Source: CAD feature listing. Evaluate the final solid. Frame: model axes, mm. A direction names the side the tool comes from. Give positions to 0.01 mm unless a question says otherwise; leave off trailing zeros. Order: outer loops, then holes, each group sorted by start corner. A loop starts at its lowest first (then second) coordinate and runs counter-clockwise, first axis right, second up.
```python
from build123d import *

# Parameters (mm, degrees)
RESSALTO_EXTRUS_O1_DEPTH = 3
RESSALTO_EXTRUS_O2_DEPTH = 1.7
ESBO_O3_R                = 1.75
RESSALTO_EXTRUS_O3_DEPTH = 2


with BuildPart() as part:
    # Esboço1 → Ressalto-extrusão1 (new body)
    with BuildSketch(Plane.XY):
        with BuildLine():
            Line((-7.992880918, 7), (-10.832226897, 4.160654021))
            Line((-10.832226897, 4.160654021), (-8.085786438, 1.414213562))
            ThreePointArc((-8.085786438, 1.414213562), (-8.085786438, -1.414213562), (-10.914213562, -1.414213562))
            Line((-10.914213562, -1.414213562), (-13.660654021, 1.332226897))
            Line((-13.660654021, 1.332226897), (-14.992880918, 0))
            Line((-14.992880918, 0), (-7.992880918, -7))
            Line((-7.992880918, -7), (-2, -7))
            Line((-2, -7), (-2, -3))
            ThreePointArc((-2, -3), (0, -1), (2, -3))
            Line((2, -3), (2, -7))
            Line((2, -7), (7.992880918, -7))
            Line((7.992880918, -7), (14.992880918, 0))
            Line((14.992880918, 0), (13.660654021, 1.332226897))
            Line((13.660654021, 1.332226897), (10.914213562, -1.414213562))
            ThreePointArc((10.914213562, -1.414213562), (8.085786438, -1.414213562), (8.085786438, 1.414213562))
            Line((8.085786438, 1.414213562), (10.832226897, 4.160654021))
            Line((10.832226897, 4.160654021), (7.992880918, 7))
            Line((7.992880918, 7), (-7.992880918, 7))
        make_face()
    extrude(amount=RESSALTO_EXTRUS_O1_DEPTH)

    # Esboço2 → Ressalto-extrusão2 (add)
    with BuildSketch(Plane.XY.offset(3)):
        Polygon((-11.267766953, -1.060660172), (-8.439339828, 1.767766953), (-10.832226897, 4.160654021), (-7.992880918, 7), (7.992880918, 7), (10.832226897, 4.160654021), (8.439339828, 1.767766953), (11.267766953, -1.060660172), (13.660654021, 1.332226897), (14.992880918, 0), (7.992880918, -7), (2, -7), (2, -3.5), (-2, -3.5), (-2, -7), (-7.992880918, -7), (-14.992880918, 0), (-13.660654021, 1.332226897), align=None)
    extrude(amount=RESSALTO_EXTRUS_O2_DEPTH)

    # Esboço3 → Ressalto-extrusão3 (add)
    with BuildSketch(Plane(origin=(0, 7, 0), x_dir=(1, 0, 0), z_dir=(0, 1, 0))):
        with BuildLine():
            Line((4, -13.7), (4, -4.7))
            Line((4, -4.7), (-4, -4.7))
            Line((-4, -4.7), (-4, -13.7))
            ThreePointArc((-4, -13.7), (0, -17.7), (4, -13.7))
        make_face()
        with Locations(Location((0, -13.7, 0), (0, 0, 90))):
            Circle(ESBO_O3_R, mode=Mode.SUBTRACT)
    extrude(amount=-RESSALTO_EXTRUS_O3_DEPTH)


solid = part.part
```
1) Reachability of faces 4 (the flat face through (0, -3, 3)), 5 (the flat face through (-11.444, -3.549, 2.317)), 6 (the cylindrical face through (-8.055, -1.383, 1.479)), 7 (the flat face through (9.834, 0.373, 3.838)), 8 (the flat face through (0, -3.5, 4)) from +Z, -Z, +X, -X, +Y, -Y: full face, straight path, thin tool, end or side. Return the list, or none.
Report:
face 4: -Z, -Y
face 5: +Z, -Z, -X, -Y
face 6: -Z
face 7: +Z, -Z
face 8: +Z, -Z, -Y
2) Draft query along X for faces 1 (the flat face through (9, -1, 3)), 2 (the flat face through (14.317, 0.675, 2.317)), 3 (the flat face through (0, 7, 7)). Return one class per face: +X half, -X half, draft (parallel to the pull), parting line (faces both ways), or undercut.
Report:
face 1: undercut
face 2: +X half
face 3: draft
3) Section query C-C, the plane z = 4. Return the cut outline in (x, y), and give its area (3 significant figures).
Report:
outline: (-14.99, 0) - (-7.99, -7) - (-2, -7) - (-2, -3.5) - (2, -3.5) - (2, -7) - (7.99, -7) - (14.99, 0) - (13.66, 1.33) - (11.27, -1.06) - (8.44, 1.77) - (10.83, 4.16) - (7.99, 7) - (-7.99, 7) - (-10.83, 4.16) - (-8.44, 1.77) - (-11.27, -1.06) - (-13.66, 1.33) - close
area: 281 mm2
4) Section query B-B, the plane y = -0.5. Return the cut outline in (x, z).
Report:
outline: (-14.49, 0) - (-11.83, 0) - (-11.83, 4.7) - (-14.49, 4.7) - close; (-10.71, 3) - (-7.56, 3) - (-7.56, 0) - (7.56, 0) - (7.56, 3) - (10.71, 3) - (10.71, 4.7) - (-10.71, 4.7) - close; (11.83, 0) - (14.49, 0) - (14.49, 4.7) - (11.83, 4.7) - close
5) Section query A-A, the plane x = 0. Return the cut outline in (y, z), and give its area (4 significant figures).
Report:
outline: (-3.5, 3) - (-1, 3) - (-1, 0) - (7, 0) - (7, 11.95) - (5, 11.95) - (5, 4.7) - (-3.5, 4.7) - close; (5, 15.45) - (7, 15.45) - (7, 17.7) - (5, 17.7) - close
area: 60.85 mm2
6) Material intervals for L1, parallel to X at y = 6.15, z = 13.7; L2, parallel to Z at x = -7.25, y = 2.75; L3, parallel to Y at x = -10, z = 1.25, sorted ascending.
Report:
L1: x = -4 to -1.75, 1.75 to 4
L2: z = 0 to 4.7
L3: y = -4.99 to -1.94, 3.33 to 4.99
7) Section query D-D, the plane y = -6. Return the cut outline in (x, z).
Report:
outline: (-8.99, 0) - (-2, 0) - (-2, 4.7) - (-8.99, 4.7) - close; (2, 0) - (8.99, 0) - (8.99, 4.7) - (2, 4.7) - close
8) Pin query (flat end, axial travel): pin 1 (2 mm diameter, centred on x = 0, y = -3, fed in from -Z); pin 2 (1.5 mm diameter, centred on y = 4.5, z = 12.5, fed in from -X); pin 3 (10 mm diameter, centred on x = 5, z = 11.5, fed in from +Y); pin 4 (5.5 mm diameter, centred on x = 0, z = 13.7, fed in from -Y). Return the tip coordinate at first contact, or that it passes through.
Report:
pin 1: stops at z = 3
pin 2: stops at x = -4
pin 3: stops at y = 7
pin 4: stops at y = 5
